The model under review builds one solid part; all positions refer to its coordinate system, in mm. Face numbers are marked on the shaded views. Give positions to 0.01 mm unless a question says otherwise; leave off trailing zeros. Order: outer loops, then holes, each group sorted by start corner. A loop starts at its lowest first (then second) coordinate and runs counter-clockwise, first axis right, second up. Notation, with made-up numbers: M 87.25,85.5 L 130.25,85.5 A6 cw 130.25,96.5 Z; hole C 78.25,4.5 d8. An arc over 180 degrees is marked long. One line per question, with ' | ' between items. Start each with the question number.
1. We need section A-A on x = 16. Write out the cut boundary in (y, z).
2. We need section B-B on x = 24. Write out the cut boundary in (y, z), then the cut area to 3 significant figures.
3. Wall thickness on L1, parallel to Y at x = -16, z = 3.81; L2, parallel to Y at x = 9.25, z = 3.81; L3, parallel to X at y = 4.75, z = -4: over which ranges is each line inside the solid? List them lowest first.
4. Insertion check: P1, Ø6, axis at y = -5.5, z = 11, coming from the -X side; P2, Ø4, axis at y = 3, z = 4, coming from the +X side; P3, Ø8, axis at x = -18, z = 4.5, coming from the +Y side. Each pin has a flat end and moves straight along its axis. Give the tip position at first contact, or say it passes through.
5. The part is to be moulded in two halves that separate along Y. For the marked faces 1, 2 and 3, say which applies: +Y half, -Y half, draft (parallel to the pull), parting line (faces both ways), or undercut.
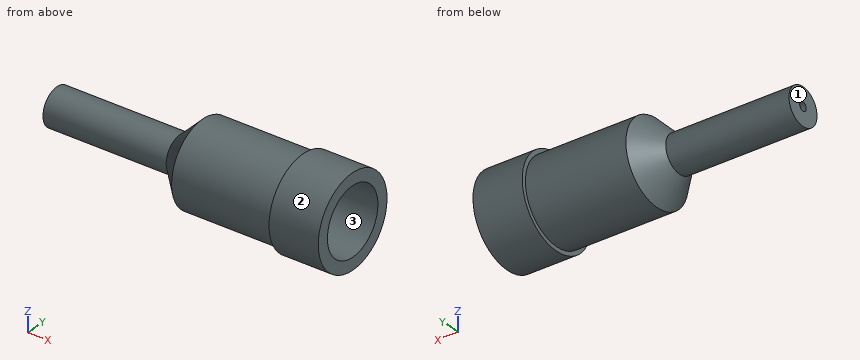
```python
from build123d import *

# Parameters (mm, degrees)
F2_S5_R     = 8.4836
F2_T6_DEPTH = 14


# Not quite as in the source:
# - a fillet or chamfer that OpenCascade refuses, or shapes differently, is made with other operations: its cross-section is extruded or revolved along the edge and cut away or added


with BuildPart() as f1:
    # F0 (on Front) → F1 (revolve)
    with BuildSketch(Plane.XZ):
        Polygon((-33.02, 0), (-2.54, 0), (-2.54, -4.6736), (17.78, -4.6736), (17.78, -5.5245), (27.94, -5.5245), (27.94, -3.048), (0, -3.048), (0, 2.921), (-33.02, 2.921), align=None)
    revolve(axis=Axis((-5.3856544969, 0, 3.81), (1, 0, 0)))

    # F2: chamfer of 5.08 on 1 edges, made by hand


with BuildPart() as f2_tool2:
    # F2_s3 → F2_t4 (revolve)
    with BuildSketch(Plane.XZ):
        Polygon((-7.62, 0), (-2.54, -5.08), (-2.54, 0), align=None)
    revolve(axis=Axis((-2.54, 0, 3.81), (1, 0, 0)))

    # F2_s5 → F2_t6 (intersect, symmetric)
    with BuildSketch(Plane.YZ.offset(-5.1)):
        with Locations((0, 3.81)):
            Circle(F2_S5_R)
    extrude(amount=F2_T6_DEPTH, both=True, mode=Mode.INTERSECT)


with BuildPart() as f1_1:
    add(f1.part)

    # F2_t1: union F2_tool2
    add(f2_tool2.part)


solid = f1_1.part
```
Entries:
1) outline: C 0,3.81 d16.97; hole C 0,3.81 d13.72
2) outline: C 0,3.81 d18.67; hole C 0,3.81 d13.72 | area: 126 mm^2
3) L1: y = -3.81 to -0.89, 0.89 to 3.81 | L2: y = -8.48 to -6.86, 6.86 to 8.48 | L3: x = 17.78 to 27.94
4) P1: stops at x = -5.38 | P2: stops at x = 0 | P3: stops at y = 3.81
5) face 1: draft | face 2: parting line | face 3: undercut
